from build123d import *

# Parameters (mm, degrees)
ESQUISSE1_R        = 0.375
ESQUISSE2_R        = 1.5
BOSS_EXTRU_1_DEPTH = 1
ESQUISSE3_R        = 2
ESQUISSE3_R_2      = 1.5
BOSS_EXTRU_2_DEPTH = 4


with BuildPart() as part:
    # Esquisse1 → Révolution1 (revolve)
    with BuildSketch(Plane.XY):
        with Locations((-0.375, 2)):
            Circle(ESQUISSE1_R)
        Polygon((-10.75, 1.5), (-1.75, 1.5), (-1.75, 1.9), (-3.75, 1.9), (-3.75, 2.5), (-4.25, 2.5), (-7.25, 1.9), (-7.25, 2.5), (-7.75, 2.5), (-10.75, 1.9), align=None)
    revolve(axis=Axis((0, 0, 0), (-1, 0, 0)))

    # Esquisse2 → Boss.-Extru.1 (add)
    with BuildSketch(Plane(origin=(-1.75, 0, 0), x_dir=(0, 0, -1), z_dir=(1, 0, 0))):
        Polygon((-2.5, -1.443375673), (-2.5, 1.443375673), (0, 2.886751346), (2.5, 1.443375673), (2.5, -1.443375673), (0, -2.886751346), align=None)
        with Locations(Location((0, 0, 0), (0, 0, 90))):
            Circle(ESQUISSE2_R, mode=Mode.SUBTRACT)
    extrude(amount=BOSS_EXTRU_1_DEPTH)

    # Esquisse3 → Boss.-Extru.2 (add)
    with BuildSketch(Plane(origin=(-0.75, 0, 0), x_dir=(0, 0, -1), z_dir=(1, 0, 0))):
        with Locations(Location((0, 0, 0), (0, 0, 270))):
            Circle(ESQUISSE3_R)
        with Locations(Location((0, 0, 0), (0, 0, 90))):
            Circle(ESQUISSE3_R_2, mode=Mode.SUBTRACT)
    extrude(amount=BOSS_EXTRU_2_DEPTH)


solid = part.part
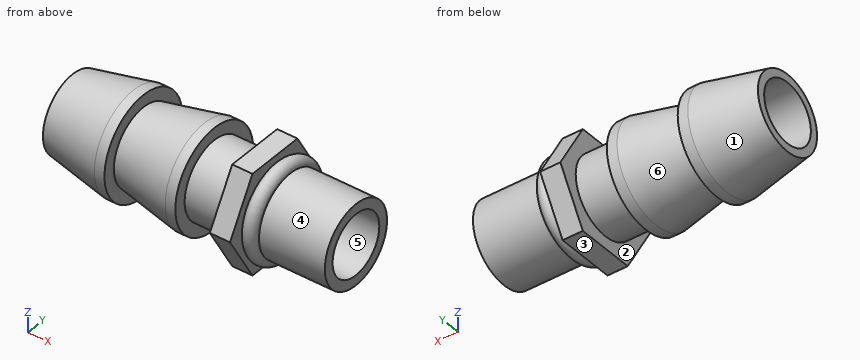
Here's how the part is built. I have some questions about the finished solid (model axes, mm). Face numbers are marked on the shaded views. A direction names the side the tool comes from. Give positions to 0.01 mm unless a question says otherwise; leave off trailing zeros. Order: outer loops, then holes, each group sorted by start corner. A loop starts at its lowest first (then second) coordinate and runs counter-clockwise, first axis right, second up. Notation, with made-up numbers: (71.25, -18) -> (100.25, -18) arc R25 ccw to (100.25, 14) -> close; hole circle Ø1 at (21.25, 80.5). An arc over 180 degrees is marked (long way). Use a Markdown table: item, result. Add a question column.
Item 1: I need wall thicknesses on line 1 (Z direction, x = -2.25, y = 0); line 2 (Z direction, x = -5.5, y = -0.9); line 3 (Y direction, x = -6.25, z = 0). Which ranges of each line are inside material? Lowest first, please.
Item 2: Will these pins go through, and if not, where does the flat tip stop? pin 1 (1 mm diameter, centred on y = 0.5, z = 0.5, fed in from -X); pin 2 (1 mm diameter, centred on y = 2, z = 0, fed in from -X); pin 3 (3 mm diameter, centred on x = -6, z = 0, fed in from -Y).
Item 3: Imagine slicing it at C-C on x = 2.75. Please give me the cut outline in (y, z), plus the area to 3 significant figures.
Item 4: If we mould it in two halves opening along X, with no side actions, what happens to the marked faces 1, 2 and 3? For each: pulls with the +X half, pulls with the -X half, needs draft (parallel to the pull), parting line crosses it, or undercut.
Item 5: For the marked faces 4, 5 and 6, which set-ups out of +Z, -Z, +X, -X, +Y, -Y let a thin tool reach every point of the face, with its end or its side?
Item 6: Imagine slicing it at B-B on x = -2.75. Please give me the cut outline in (y, z), plus the area to 3 significant figures.
Data:
| question | item | result |
|---|---|---|
| 1 | line 1 | z = -1.9 to -1.5, 1.5 to 1.9 |
| 1 | line 2 | z = -2.06 to -1.2, 1.2 to 2.06 |
| 1 | line 3 | y = -2.1 to -1.5, 1.5 to 2.1 |
| 2 | pin 1 | passes through |
| 2 | pin 2 | stops at x = -10.75 |
| 2 | pin 3 | stops at y = -2.5 |
| 3 | outline | circle Ø4 at (0, 0); hole circle Ø3 at (0, 0) |
| 3 | area | 5.50 mm² |
| 4 | face 1 | pulls with the -X half |
| 4 | face 2 | undercut |
| 4 | face 3 | needs draft |
| 5 | face 4 | +X |
| 5 | face 5 | +X, -X |
| 5 | face 6 | none |
| 6 | outline | circle Ø3.8 at (0, 0); hole circle Ø3 at (0, 0) |
| 6 | area | 4.27 mm² |
